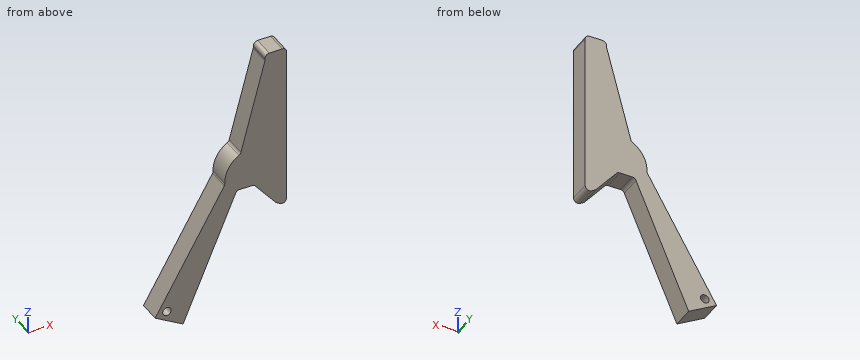
from build123d import *

# Parameters (mm, degrees)
SKETCH1_R           = 2
BOSS_EXTRUDE1_DEPTH = 10
FILLET1_R           = 2


with BuildPart() as part:
    # Sketch1 → Boss-Extrude1 (new body)
    with BuildSketch(Plane(origin=(0, 0, 0), x_dir=(1, 0, 0), z_dir=(0, 1, 0))):
        with BuildLine():
            Line((13.99715319, 15.809310821), (1.006772133, 8.309310821))
            Line((1.006772133, 8.309310821), (33.506772133, -47.982340425))
            ThreePointArc((33.506772133, -47.982340425), (35.087704929, -55.582092399), (40.71773761, -60.926090021))
            Line((40.71773761, -60.926090021), (52.173142167, -104.443600363))
            Line((52.173142167, -104.443600363), (52.173142167, -107.443600363))
            Line((52.173142167, -107.443600363), (62.173142167, -107.443600363))
            Line((62.173142167, -107.443600363), (62.173142167, -27.443600363))
            Line((62.173142167, -27.443600363), (57.158909288, -30.738667683))
            Line((57.158909288, -30.738667683), (47.003945413, -43.1029998))
            Line((47.003945413, -43.1029998), (39.003945413, -43.1029998))
            Line((39.003945413, -43.1029998), (13.99715319, 15.809310821))
        make_face()
        with Locations(Location((6.470873748, 6.845209206, 0), (0, 0, 270))):
            Circle(SKETCH1_R, mode=Mode.SUBTRACT)
    extrude(amount=BOSS_EXTRUDE1_DEPTH)

    # Fillet1
    fillet1_edges = [part.edges().sort_by_distance(p)[0] for p in [
        (39.003945413, 5, 43.1029998),
        (47.003945413, 5, 43.1029998),
        (57.158909288, 5, 30.738667683),
        (62.173142167, 5, 27.443600363),
        (62.173142167, 5, 107.443600363),
        (52.173142167, 5, 107.443600363),
        (52.173142167, 5, 104.443600363),
        (40.71773761, 5, 60.926090021),
        (33.506772133, 5, 47.982340425),
    ]]
    fillet(fillet1_edges, radius=FILLET1_R)


solid = part.part
For this review, take the finished solid that the model builds, in its own axes (mm). Coordinates: 2 decimals unless noted, no trailing zeros. Loops run counter-clockwise (first coordinate to the right, second up) from the corner with the lowest first, then second, coordinate; pieces in that order, holes last. Notation, with made-up numbers: (-1.5, 57.25) - (22.5, 57.25) arc R14 ccw to (22.5, 76.25) - close; hole circle Ø10 at (52.5, 35). An arc over 180 degrees is marked (long way). Return JSON: item names as keys, results as strings.
Item 1: Take a section at D-D (z = 67). Give the boundary of the cut face in (x, y), then the cut area to 3 significant figures.
Determined:
{"outline": "(42.32, 0) - (62.17, 0) - (62.17, 10) - (42.32, 10) - close", "area": "199 mm2"}
Item 2: Take a section at C-C (x = 51). Give the boundary of the cut face in (y, z), then the cut area to 3 significant figures.
Determined:
{"outline": "(0, 38.24) - (10, 38.24) - (10, 99.99) - (0, 99.99) - close", "area": "617 mm2"}
Item 3: Take a section at B-B (y = 7.5). Give the boundary of the cut face in (x, z).
Determined:
{"outline": "(1.01, -8.31) - (14, -15.81) - (38.49, 41.88) arc R2 cw to (40.33, 43.1) - (46.06, 43.1) arc R2 cw to (47.6, 42.37) - (56.97, 30.97) arc R2 ccw to (57.41, 30.57) - (59.07, 29.48) arc R2 ccw to (62.17, 31.15) - (62.17, 105.44) arc R2 ccw to (60.17, 107.44) - (54.17, 107.44) arc R2 ccw to (52.17, 105.44) - (52.17, 104.7) arc R2 cw to (52.11, 104.19) - (40.94, 61.77) arc R2 cw to (40, 60.54) arc R13 ccw to (33.46, 48.56) arc R2 cw to (33.2, 47.45) - close; hole circle Ø4 at (6.47, -6.85)"}
Item 4: For line 1 (X direction, y = 1.5, z = 6); line 2 (X direction, y = 5.75, z = 7); line 3 (Z direction, x = 38, y = 9), list the stretches that pass through material, from the lowest coordinate up.
Determined:
{"line 1": "x = 9.27 to 23.25", "line 2": "x = 9.85 to 23.68", "line 3": "z = 40.74 to 59.14"}
Item 5: Take a section at A-A (z = 39). Give the boundary of the cut face in (x, y).
Determined:
{"outline": "(28.32, 0) - (37.26, 0) - (37.26, 10) - (28.32, 10) - close; (50.37, 0) - (62.17, 0) - (62.17, 10) - (50.37, 10) - close"}
Item 6: Insertion check: pin 1 (5 mm diameter, centred on x = 56, y = 7.5, fed in from -Z); pin 2 (6 mm diameter, centred on y = 6, z = 7.5, fed in from -X); pin 3 (4.5 mm diameter, centred on x = 44.5, y = 3, fed in from -Z); pin 4 (3.5 mm diameter, centred on x = 6.47, z = -6.85, fed in from +Y). Each pin has a flat end and moves straight along its axis. Give the tip position at first contact, or say it passes through.
Determined:
{"pin 1": "stops at z = 29.86", "pin 2": "stops at x = 8.4", "pin 3": "stops at z = 42.98", "pin 4": "passes through"}
